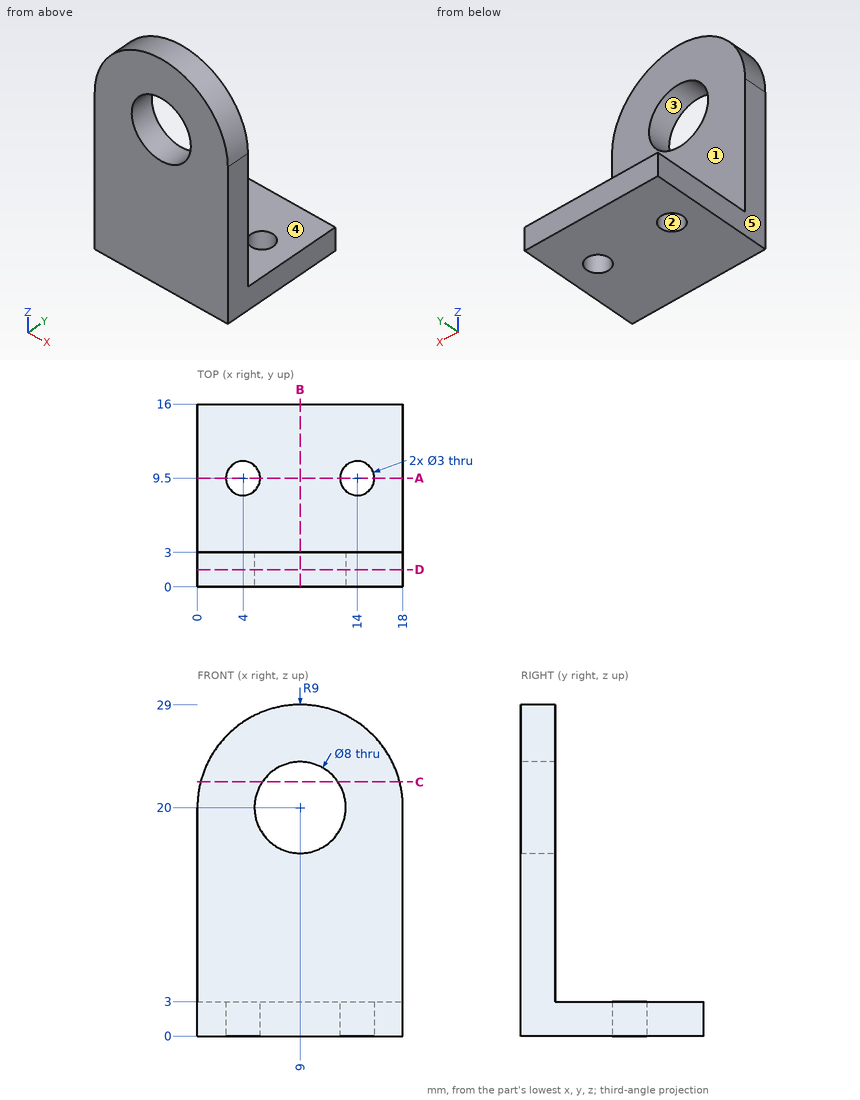
Design review of the part shown in the three views and the two pictorial views. Dimensions are in mm from the part's minimum x, y and z. A direction names the side the tool comes from. Round coordinates to 2 decimals unless told otherwise and drop trailing zeros. Write each loop counter-clockwise with the first axis right and the second up, starting at its lowest first coordinate (ties: lowest second). Pieces come first, ordered by that corner, then holes. Notation, with made-up numbers: (46, 76.5) -> (64, 76.5) arc R30 cw to (64, 105.5) -> close; hole circle Ø8 at (43, 86.25). An arc over 180 degrees is marked (long way). One line per question, with ' | ' between items. Start each with the question number.
1) Wall thickness on line 1 along Y through (x, z) = (14, 1.2); line 2 along X through (y, z) = (1.75, 20); line 3 along Z through (x, y) = (11.5, 12.5): over which ranges is each line inside the solid? List them lowest first.
2) Add section A-A (y = 9.5). Write out the cut boundary in (x, z), and give its area (3 significant figures).
3) For pin 1 Ø6.5 at (x, y) = (13, 12.5) entering from +Z; pin 2 Ø5.5 at (x, z) = (4.5, 20) entering from +Y, all flat-tipped, find the tip position at first contact; note any pin that passes through.
4) Add section D-D (y = 1.5). Write out the cut boundary in (x, z).
5) Add section B-B (x = 9). Write out the cut boundary in (y, z).
6) Add section C-C (z = 22.25). Write out the cut boundary in (x, y).
7) Mouldability with a two-part tool opening along Y and no side actions: class the marked faces 1, 2 and 3 as +Y half, -Y half, draft (parallel to the pull), parting line (faces both ways), or undercut.
8) Machinability: for the marked faces 4 and 5, which of the approach directions +Z, -Z, +X, -X, +Y, -Y give a long, thin tool a straight path to every point of the face, cutting with its end or side? Answer none if there is none.
Reported:
1) line 1: y = 0 to 8, 11 to 16 | line 2: x = 0 to 5, 13 to 18 | line 3: z = 0 to 3
2) outline: (0, 0) -> (2.5, 0) -> (2.5, 3) -> (0, 3) -> close; (5.5, 0) -> (12.5, 0) -> (12.5, 3) -> (5.5, 3) -> close; (15.5, 0) -> (18, 0) -> (18, 3) -> (15.5, 3) -> close | area: 36.0 mm²
3) pin 1: stops at z = 3 | pin 2: stops at y = 3
4) outline: (0, 0) -> (18, 0) -> (18, 20) arc R9 ccw to (0, 20) -> close; hole circle Ø8 at (9, 20)
5) outline: (0, 0) -> (16, 0) -> (16, 3) -> (3, 3) -> (3, 16) -> (0, 16) -> close; (0, 24) -> (3, 24) -> (3, 29) -> (0, 29) -> close
6) outline: (0.29, 0) -> (5.69, 0) -> (5.69, 3) -> (0.29, 3) -> close; (12.31, 0) -> (17.71, 0) -> (17.71, 3) -> (12.31, 3) -> close
7) face 1: +Y half | face 2: undercut | face 3: draft
8) face 4: +Z, +X, -X, +Y | face 5: +Z, -Z, -X, +Y, -Y
